Can you work these out from the model? Positions are in its coordinate system, mm. Face numbers are marked on the shaded views. A direction names the side the tool comes from. Coordinates: 2 decimals unless noted, no trailing zeros. Loops run counter-clockwise (first coordinate to the right, second up) from the corner with the lowest first, then second, coordinate; pieces in that order, holes last.
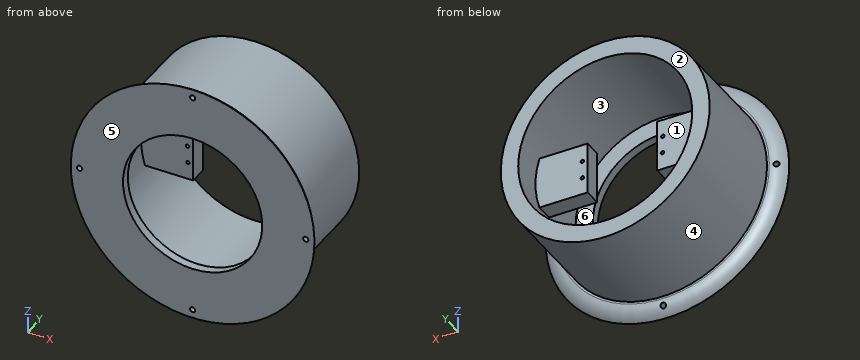
```python
from build123d import *

# Parameters (mm, degrees)
SKETCH1_R                = 60
BOSS_EXTRUDE1_DEPTH      = 60
SHELL1_T                 = -10
SKETCH2_R                = 70
BOSS_EXTRUDE2_DEPTH      = 5
SKETCH5_R                = 40
CUT_EXTRUDE4_DEPTH       = 5
FILLET1_R                = 10
BOSS_EXTRUDE4_DEPTH      = 55
BOSS_EXTRUDE4_DEPTH_BACK = 54
SKETCH7_W                = 30
SKETCH7_H                = 10
SKETCH8_W                = 40
SKETCH8_H                = 32
CUT_EXTRUDE6_DEPTH       = 55
SKETCH9_R                = 1
CUT_EXTRUDE7_DEPTH       = 55
SKETCH10_R               = 1.5
CUT_EXTRUDE8_DEPTH       = 30


with BuildPart() as part:
    # Sketch1 → Boss-Extrude1 (new body)
    with BuildSketch(Plane(origin=(0, 0, 0), x_dir=(1, 0, 0), z_dir=(0, 1, 0))):
        with Locations(Location((0, 0, 0), (0, 0, 270))):
            Circle(SKETCH1_R)
    extrude(amount=BOSS_EXTRUDE1_DEPTH)

    # Shell1
    shell1_openings = [part.faces().sort_by_distance(p)[0] for p in [
        (0, 60, 0),
        (0, 0, 0),
    ]]
    offset(amount=SHELL1_T, openings=shell1_openings, kind=Kind.INTERSECTION)

    # Sketch2 → Boss-Extrude2 (add)
    with BuildSketch(Plane(origin=(0, 0, 0), x_dir=(1, 0, 0), z_dir=(0, 1, 0))):
        with Locations(Location((0, 0, 0), (0, 0, 270))):
            Circle(SKETCH2_R)
    extrude(amount=-BOSS_EXTRUDE2_DEPTH)

    # Sketch5 → Cut-Extrude4 (cut)
    with BuildSketch(Plane(origin=(0, 0, 0), x_dir=(1, 0, 0), z_dir=(0, 1, 0))):
        with Locations(Location((0, 0, 0), (0, 0, 270))):
            Circle(SKETCH5_R)
    extrude(amount=-CUT_EXTRUDE4_DEPTH, mode=Mode.SUBTRACT)

    # Fillet1
    # the kernel refuses this fillet: 10 mm, written as the material it takes off along each edge
    with BuildSketch(Plane(origin=(0, 0, 0), x_dir=(0, 0, 1), z_dir=(-1, 0, 0))) as fillet1_piece_1:
        with BuildLine():
            CenterArc((61.339745962, -10), FILLET1_R, 30, 60)
            Line((61.339745962, 0), (61.339745962, 0.2))
            Line((61.339745962, 0.2), (70, 0.2))
            Line((70, 0.2), (70.2, 0))
            ThreePointArc((70.2, 0), (70.2, -2.5), (70.173205081, -4.9))
            Line((70.173205081, -4.9), (70, -5))
        make_face()
    revolve(axis=Axis((0, 0, 0), (0, 1, 0)), mode=Mode.SUBTRACT)

    # Sketch7 → Boss-Extrude4 (add, two sides: drawn at the far end of the back side and taken through both)
    with BuildSketch(Plane(origin=(0, 0, 0), x_dir=(0, 0, -1), z_dir=(1, 0, 0)).offset(-BOSS_EXTRUDE4_DEPTH_BACK)):
        with Locations((0, 37)):
            Rectangle(SKETCH7_W, SKETCH7_H)
    extrude(amount=BOSS_EXTRUDE4_DEPTH + BOSS_EXTRUDE4_DEPTH_BACK)

    # Sketch8 → Cut-Extrude6 (cut)
    with BuildSketch(Plane(origin=(0, 0, 0), x_dir=(1, 0, 0), z_dir=(0, 1, 0))):
        Rectangle(SKETCH8_W, SKETCH8_H)
    extrude(amount=CUT_EXTRUDE6_DEPTH, mode=Mode.SUBTRACT)

    # Sketch9 → Cut-Extrude7 (cut)
    with BuildSketch(Plane(origin=(0, 0, 0), x_dir=(1, 0, 0), z_dir=(0, 1, 0))):
        with Locations(Location((-23, 5, 0), (0, 0, 90))):
            Circle(SKETCH9_R)
        with Locations(Location((-23.236551587, -5, 0), (0, 0, 90))):
            Circle(SKETCH9_R)
        with Locations(Location((23, 5, 0), (0, 0, 90))):
            Circle(SKETCH9_R)
        with Locations(Location((23, -5, 0), (0, 0, 90))):
            Circle(SKETCH9_R)
    extrude(amount=CUT_EXTRUDE7_DEPTH, mode=Mode.SUBTRACT)

    # Sketch10 → Cut-Extrude8 (cut)
    with BuildSketch(Plane(origin=(0, 0, 0), x_dir=(1, 0, 0), z_dir=(0, 1, 0))):
        with Locations(Location((0, 65, 0), (0, 0, 270))):
            Circle(SKETCH10_R)
        with Locations(Location((65, 0, 0), (0, 0, 270))):
            Circle(SKETCH10_R)
        with Locations(Location((0, -65, 0), (0, 0, 270))):
            Circle(SKETCH10_R)
        with Locations(Location((-65, 0, 0), (0, 0, 270))):
            Circle(SKETCH10_R)
    extrude(amount=-CUT_EXTRUDE8_DEPTH, mode=Mode.SUBTRACT)


solid = part.part
```
Item 1: Suppose I cut it at B-B, the plane x = 33.5. Count the separate pieces of the cut face and the enclosed holes in it, plus the area to 3 significant figures.
Results are:
separate pieces: 3
enclosed holes: 0
area: 2,190 mm2
Item 2: I'm going to push flat-ended pins straight in: P1, Ø2, axis at y = 38.5, z = 11.5, coming from the -X side; P2, Ø11, axis at y = 38, z = 7, coming from the -X side; P3, Ø8, axis at x = 36, y = 39.5, coming from the +Z side; P4, Ø1.8, axis at x = 0, z = -65, coming from the +Y side. Where does each tip first touch, or does it pass through?
Results are:
P1: stops at x = -59.07
P2: stops at x = -59.98
P3: stops at z = 50.75
P4: passes through
Item 3: I need wall thicknesses on line 1 along X through (y, z) = (-1, 0); line 2 along X through (y, z) = (-2.6, 0); line 3 along Y through (x, z) = (-45, 14). Which ranges of each line are inside material? Lowest first, please.
Results are:
line 1: x = -63.5 to -40, 40 to 63.5
line 2: x = -68.07 to -66.5, -63.5 to -40, 40 to 63.5, 66.5 to 68.07
line 3: y = -5 to 0, 32 to 42
Item 4: On a 3-axis mill with a long thin cutter (end or side, diameter ignored), from which of +Z, -Z, +X, -X, +Y, -Y can I reach the whole of each face in a straight line? I mean the marked faces 1, 2 and 3. Say none if no direction works.
Results are:
face 1: +Y
face 2: +Z, -Z, +X, -X, +Y
face 3: none
Item 5: Suppose I cut it at A-A, the plane y = 56. Please give me the cut outline in (x, z), plus the area to 3 significant figures.
Results are:
outline: circle Ø120 at (0, 0); hole circle Ø100 at (0, 0)
area: 3,460 mm2
Item 6: We'd pull the mould along X, two halves only. Please class the marked faces 4, 5 and 6: +X half, -X half, draft (parallel to the pull), parting line (faces both ways), or undercut.
Results are:
face 4: parting line
face 5: draft
face 6: undercut
